```python
from build123d import *

# Parameters (mm, degrees)
F1_DEPTH = 63.5
F0_W     = 35.9624676678
F0_H     = 20.9170691669
F2_DEPTH = 25.4
F3_DEPTH = 7.9375
F5_R     = 6.35


with BuildPart() as f1:
    # F0 (on Top) → F1 (new body, symmetric)
    with BuildSketch(Plane.XY):
        Polygon((42.8987257183, 28.2148495317), (-63.5203495622, 28.2148495317), (-63.5203495622, -24.0786485374), (63.8157948852, -24.0786485374), (63.8157948852, 28.2148495317), align=None)
    extrude(amount=F1_DEPTH, both=True)

    # F0 (on Top) → F2 (join, symmetric)
    with BuildSketch(Plane.XY):
        with BuildLine():
            Line((42.8987257183, 50.6685562432), (42.8987257183, 28.2148495317))
            Line((42.8987257183, 28.2148495317), (63.8157948852, 28.2148495317))
            Line((63.8157948852, 28.2148495317), (63.8157948852, 50.6685562432))
            ThreePointArc((63.8157948852, 50.6685562432), (68.5286535357, 61.8676195433), (79.8310190439, 66.3270577788))
            Line((79.8310190439, 66.3270577788), (93.0647104979, 66.3270577788))
            Line((93.0647104979, 66.3270577788), (93.0647104979, 87.2441269457))
            Line((93.0647104979, 87.2441269457), (80.017371915, 87.2441269457))
            add(Edge.make_bspline(
                [(78.7551044312, 87.2409507038), (79.1779792996, 87.2440139811), (79.5987547257, 87.2450791343), (80.017371915, 87.2441269457)],
                knots=[153.9975424007, 153.9975424007, 153.9975424007, 153.9975424007, 155.2015885192, 155.2015885192, 155.2015885192, 155.2015885192], degree=3))
            ThreePointArc((78.7551044312, 87.2409507038), (53.3581999175, 76.2772458377), (42.8987257183, 50.6685562432))
        make_face()
        with Locations((111.0459443317, 76.7855923623)):
            Rectangle(F0_W, F0_H)
    extrude(amount=F2_DEPTH, both=True)

    # F0 (on Top) → F3 (join, symmetric)
    with BuildSketch(Plane.XY):
        with BuildLine():
            add(Edge.make_bspline(
                [(-63.5203495622, 28.2148495317), (-63.7598756137, 53.7712109703), (24.6693933614, 86.8491574209), (78.7551044312, 87.2409507038)],
                knots=[0, 0, 0, 0, 153.9975424007, 153.9975424007, 153.9975424007, 153.9975424007], degree=3))
            Line((-63.5203495622, 28.2148495317), (42.8987257183, 28.2148495317))
            Line((42.8987257183, 28.2148495317), (42.8987257183, 50.6685562432))
            ThreePointArc((42.8987257183, 50.6685562432), (53.3581999175, 76.2772458377), (78.7551044312, 87.2409507038))
        make_face()
    extrude(amount=F3_DEPTH, both=True)

    # F0 (on Top) → F4 (revolve)
    with BuildSketch(Plane.XY):
        Polygon((129.0271781656, 93.8032977283), (129.0271781656, 87.2441269457), (129.0271781656, 66.3270577788), (129.0271781656, 50.6685562432), (162.7893596888, 50.6685562432), (162.7893596888, 93.8032977283), align=None)
    revolve(axis=Axis((129.0271781656, 72.2359269857, 0), (0, 1, 0)))

    # F5
    f5_edges = [f1.edges().sort_by_distance(p)[0] for p in [
        (-63.52035, 2.0681, -63.5),
        (63.815795, 2.0681, -63.5),
        (-63.52035, 2.0681, 63.5),
        (63.815795, 2.0681, 63.5),
    ]]
    fillet(f5_edges, radius=F5_R)


solid = f1.part
```
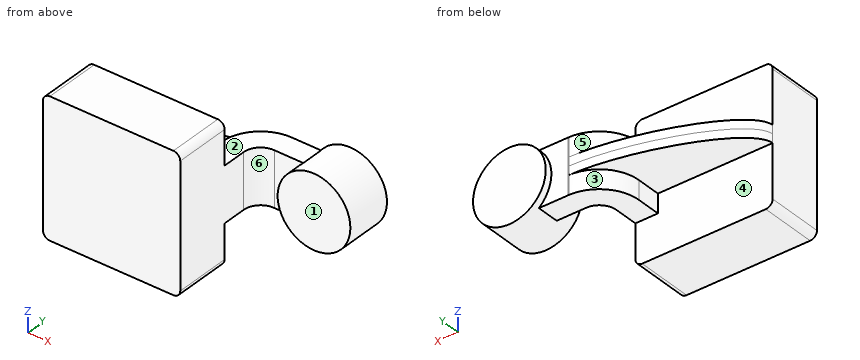
The listing builds one solid part. Answer for the finished solid, in the listing's coordinates (mm). Face numbers are marked on the shaded views. A direction names the side the tool comes from. Give positions to 0.01 mm unless a question says otherwise; leave off trailing zeros. Order: outer loops, then holes, each group sorted by start corner. A loop starts at its lowest first (then second) coordinate and runs counter-clockwise, first axis right, second up. Notation, with made-up numbers: (51, -25.75) - (82, -25.75) arc R20 cw to (82, -2.75) - close; hole circle Ø9 at (35, -12). An arc over 180 degrees is marked (long way). Answer in a Markdown table with one row per item. Add a question column.
Q1. The part is cut by section B-B (x = 103). Determine the outline of the cut face in (y, z).
Q2. Given P1, Ø12, axis at x = 27, z = 47.5, coming from the +Y side; P2, Ø1, axis at y = 37, z = -7.5, coming from the -X side; P3, Ø14, axis at y = 41.5, z = 17.5, coming from the -X side; P4, Ø6, axis at x = -24.5, y = 68, coming from the -Z side, each flat-ended and moving along its own axis, determine where each tip first touches the part or whether it passes through.
Q3. Find the intervals of material crossed by line 1 along Y through (x, z) = (14.5, -57.5); line 2 along Y through (x, z) = (120.5, -30.5); line 3 along Z through (x, y) = (128.5, 67.5), in increasing order. Write a range as [from, to].
Q4. For a pull along X with two mould halves and no side action, classify the marked faces 4, 5 and 6 as released by +X, released by -X, zero draft, split by the parting line, or undercut.
Q5. The part is cut by section A-A (y = -2.5). Determine the outline of the cut face in (x, z), then the cut area to 3 significant figures.
Q6. Which of the six approach directions +Z, -Z, +X, -X, +Y, -Y give full straight-line access (tool end or side, diameter ignored) to the marked faces 1, 2 and 3?
Q7. The part is cut by section C-C (z = -51). Determine the outline of the cut face in (x, y).
Determined:
| question | item | result |
|---|---|---|
| 1 | outline | (50.67, -21.51) - (66.33, -21.51) - (66.33, -25.4) - (87.24, -25.4) - (87.24, -21.51) - (93.8, -21.51) - (93.8, 21.51) - (87.24, 21.51) - (87.24, 25.4) - (66.33, 25.4) - (66.33, 21.51) - (50.67, 21.51) - close |
| 2 | P1 | stops at y = 28.21 |
| 2 | P2 | stops at x = -60.78 |
| 2 | P3 | stops at x = 42.9 |
| 2 | P4 | passes through |
| 3 | line 1 | y = [-24.08, 28.21] |
| 3 | line 2 | y = [50.67, 93.8] |
| 3 | line 3 | z = [-33.76, 33.76] |
| 4 | face 4 | zero draft |
| 4 | face 5 | released by -X |
| 4 | face 6 | undercut |
| 5 | outline | (-63.52, -57.15) arc R6.35 ccw to (-57.17, -63.5) - (57.47, -63.5) arc R6.35 ccw to (63.82, -57.15) - (63.82, 57.15) arc R6.35 ccw to (57.47, 63.5) - (-57.17, 63.5) arc R6.35 ccw to (-63.52, 57.15) - close |
| 5 | area | 16,100 mm² |
| 6 | face 1 | +Z, -Z, +X, -Y |
| 6 | face 2 | +Z, -X, +Y |
| 6 | face 3 | -Z, -X, +Y |
| 7 | outline | (-63.52, -24.08) - (63.82, -24.08) - (63.82, 28.21) - (-63.52, 28.21) - close |
